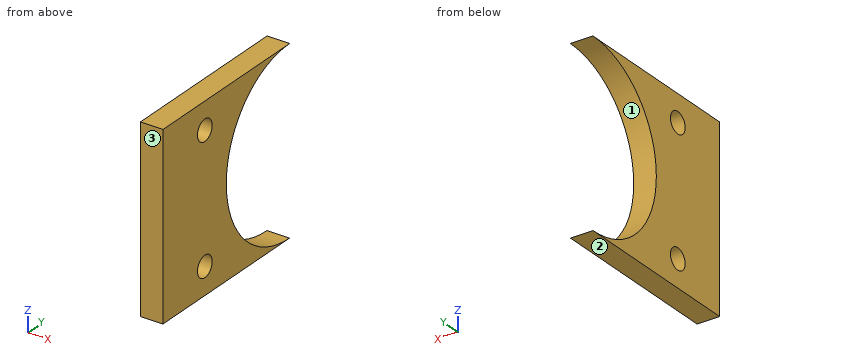
from build123d import *

# Parameters (mm, degrees)
BOSS_EXTRUDE1_DEPTH = 3.175
SKETCH6_R           = 1.473196931
CUT_EXTRUDE2_DEPTH  = 19.238986403


with BuildPart() as part:
    # Sketch1 → Boss-Extrude1 (new body)
    with BuildSketch(Plane(origin=(0, 0, 0), x_dir=(0, 0, -1), z_dir=(1, 0, 0))):
        with BuildLine():
            Line((-12.7, -12.7), (12.7, -12.7))
            Line((12.7, -12.7), (12.7, 12.7))
            ThreePointArc((12.7, 12.7), (0, 0), (-12.7, 12.7))
            Line((-12.7, 12.7), (-12.7, -12.7))
        make_face()
    extrude(amount=BOSS_EXTRUDE1_DEPTH)

    # Sketch6 → Cut-Extrude2 (cut, symmetric)
    with BuildSketch(Plane.ZY):
        with Locations((-8.889941847, -4.308950185)):
            Circle(SKETCH6_R)
    cut_extrude2 = extrude(amount=CUT_EXTRUDE2_DEPTH, both=True, mode=Mode.SUBTRACT)

    # Mirror2: Cut-Extrude2 across plane
    add(cut_extrude2.mirror(Plane.XY), mode=Mode.SUBTRACT)


solid = part.part
The listing builds one solid part. Answer for the finished solid, in the listing's coordinates (mm). Face numbers are marked on the shaded views. Round coordinates to 2 decimals unless told otherwise and drop trailing zeros. Order: outer loops, then holes, each group sorted by start corner. A loop starts at its lowest first (then second) coordinate and runs counter-clockwise, first axis right, second up. Notation, with made-up numbers: (60.5, 72) -> (89.5, 72) arc R21 cw to (89.5, 104) -> close; hole circle Ø3 at (-32, 11). An arc over 180 degrees is marked (long way). Put each result on its own line as item: value.
Q1. Section A-A, the plane y = 6 is taken. Write down the section's boundary in (x, z) (3 decimals).
Results list:
outline: (0, -12.7) -> (3.175, -12.7) -> (3.175, -10.789) -> (0, -10.789) -> close; (0, 10.789) -> (3.175, 10.789) -> (3.175, 12.7) -> (0, 12.7) -> close
Q2. Determine the mould class of the marked faces 1, 2 and 3 for opening direction Z: pulls with the +Z half, pulls with the -Z half, needs draft (parallel to the pull), parting line crosses it, or undercut.
Results list:
face 1: undercut
face 2: pulls with the -Z half
face 3: needs draft
Q3. Each of these flat-tipped pins is pushed along its axis until it touches: P1, Ø4.5, axis at y = -4.31, z = -8.89, coming from the -X side; P2, Ø1.5, axis at x = 2.5, z = 9.5, coming from the +Y side. Where does it stop, or does it pass through?
Results list:
P1: x = 0
P2: y = 5.2
Q4. Section C-C, the plane x = 2.65 is taken. Write down the section's boundary in (y, z).
Results list:
outline: (-12.7, -12.7) -> (12.7, -12.7) arc R12.7 cw to (12.7, 12.7) -> (-12.7, 12.7) -> close; hole circle Ø2.95 at (-4.31, -8.89); hole circle Ø2.95 at (-4.31, 8.89)
Q5. Section B-B, the plane z = -8.5 is taken. Write down the section's boundary in (x, y) (3 decimals).
Results list:
outline: (0, -12.7) -> (3.175, -12.7) -> (3.175, -5.73) -> (0, -5.73) -> close; (0, -2.888) -> (3.175, -2.888) -> (3.175, 3.264) -> (0, 3.264) -> close
Q6. Consider line 1 along Z through (x, y) = (0.25, -3.5); line 2 along Z through (x, y) = (1.8, -5.5); line 3 along Z through (x, y) = (0.5, 6.5). Determine where each line is inside the solid, lowest interval first.
Results list:
line 1: -12.7 to -10.12, -7.66 to 7.66, 10.12 to 12.7
line 2: -12.7 to -9.76, -8.02 to 8.02, 9.76 to 12.7
line 3: -12.7 to -11.08, 11.08 to 12.7
Q7. Section D-D, the plane z = 0 is taken. Write down the section's boundary in (x, y) (3 decimals), and give its area (3 significant figures).
Results list:
outline: (0, -12.7) -> (3.175, -12.7) -> (3.175, 0) -> (0, 0) -> close
area: 40.3 mm^2
